Geometry check sheet. Reference: the model listing, model coordinates, mm. A direction names the side the tool comes from. Give positions to 0.01 mm unless a question says otherwise; leave off trailing zeros. Write each loop counter-clockwise with the first axis right and the second up, starting at its lowest first coordinate (ties: lowest second). Pieces come first, ordered by that corner, then holes.
(1) Cross-section at C-C (x = 43). Record the boundary of the cut face in (y, z), and give its area (3 significant figures).
(2) Depth check by flat-ended pin: P1, Ø2, axis at y = 2, z = -41, coming from the -X side; P2, Ø5, axis at x = 64.5, z = -31.5, coming from the -Y side; P3, Ø4, axis at x = 79, z = 45, coming from the -Y side; P4, Ø3.5, axis at x = -79, z = -45.5, coming from the +Y side. Enter the tip coordinate at first touch or a pass-through.
(3) Tool access check on faces 1 (the cylindrical face through (75, 1, 42)), 2 (the cylindrical face through (79.46, 2.92, -48.47)), 3 (the cylindrical face through (-77.3, 0.64, 45.07)). Record the directions out of +Z, -Z, +X, -X, +Y, -Y that give a thin tool (end or side, any length) a straight path to the whole face; none if there is none.
(4) Mould release check, pull along X, two halves, no side actions. Record for faces 4 (the flat face through (-77, 1.3, 46)), 5 (the flat face through (-84, 2, -34)), 6 (the flat face through (1, 2, -50)), 7 (the flat face through (84, 2, -34)): +X half, -X half, draft (parallel to the pull), parting line (faces both ways), or undercut.
(5) Cross-section at B-B (z = -6). Record the boundary of the cut face in (x, y), and give its area (3 significant figures).
(6) Thickness scan on line 1 along Z through (x, y) = (79, 2.6); line 2 along X through (y, z) = (2.9, -45); line 3 along Z through (x, y) = (9, 1.45). Record the ranges inside material, lowest first.
(7) Cross-section at A-A (y = 3.5). Record the boundary of the cut face in (x, z).
```python
from build123d import *

# Parameters (mm, degrees)
SKIZZE1_W                                            = 89
SKIZZE1_H                                            = 50
AUFSATZ_LINEAR_AUSTRAGEN1_DEPTH                      = 4.5
SKIZZE3_W                                            = 16
SKIZZE3_H                                            = 12
SCHNITT_LINEAR_AUSTRAGEN2_DEPTH                      = 5.5
VERRUNDUNG1_R                                        = 2
LINEARES_MUSTER1_COUNT                               = 3
LINEARES_MUSTER1_PITCH                               = 16
LINEARES_MUSTER1_COUNT_DIR2                          = 4
LINEARES_MUSTER1_PITCH_DIR2                          = 20
VERRUNDUNG1_OF_LINEARES_MUSTER1_R                    = 2
SKIZZE2_R                                            = 5
AUFSATZ_LINEAR_AUSTRAGEN2_DEPTH                      = 4.5
STIRNSENKUNG_F_R_M3_FLACHKOPFSCHRAUBE_MI_D           = 3.4
STIRNSENKUNG_F_R_M3_FLACHKOPFSCHRAUBE_MI_CBORE_D     = 7
STIRNSENKUNG_F_R_M3_FLACHKOPFSCHRAUBE_MI_CBORE_DEPTH = 3.2
VERRUNDUNG3_R                                        = 3
SCHNITT_LINEAR_AUSTRAGEN3_DEPTH                      = 1.5
AUFSATZ_LINEAR_AUSTRAGEN3_DEPTH                      = 3
SKIZZE8_W                                            = 10
SKIZZE8_H                                            = 35
SCHNITT_LINEAR_AUSTRAGEN4_DEPTH                      = 5.5
VERRUNDUNG4_R                                        = 2


with BuildPart() as part:
    # Skizze1 → Aufsatz-Linear austragen1 (new body)
    with BuildSketch(Plane(origin=(0, 0, 0), x_dir=(1, 0, 0), z_dir=(0, 1, 0))):
        with Locations((-44.5, 25)):
            Rectangle(SKIZZE1_W, SKIZZE1_H)
    extrude(amount=AUFSATZ_LINEAR_AUSTRAGEN1_DEPTH)

    # Skizze3 → Schnitt-Linear austragen2 (cut, through all)
    with BuildSketch(Plane(origin=(0, 4.5, 0), x_dir=(1, 0, 0), z_dir=(0, 1, 0))):
        with Locations((-11, 9)):
            Rectangle(SKIZZE3_W, SKIZZE3_H)
    schnitt_linear_austragen2 = extrude(amount=-SCHNITT_LINEAR_AUSTRAGEN2_DEPTH, mode=Mode.SUBTRACT)

    # Verrundung1
    verrundung1_edges = [part.edges().sort_by_distance(p)[0] for p in [
        (-3, 2.25, -15),
        (-3, 2.25, -3),
        (-19, 2.25, -3),
        (-19, 2.25, -15),
    ]]
    fillet(verrundung1_edges, radius=VERRUNDUNG1_R)

    # Lineares Muster1: Schnitt-Linear austragen2 3 × 4
    with Locations(*[(-j * LINEARES_MUSTER1_PITCH_DIR2, 0, -i * LINEARES_MUSTER1_PITCH) for i in range(LINEARES_MUSTER1_COUNT) for j in range(LINEARES_MUSTER1_COUNT_DIR2) if (i, j) != (0, 0)]):
        add(schnitt_linear_austragen2, mode=Mode.SUBTRACT)

    # Verrundung1 of Lineares Muster1
    verrundung1_of_lineares_muster1_edges = [part.edges().sort_by_distance(p)[0] for p in [
        (-23, 2.25, -15),
        (-23, 2.25, -3),
        (-39, 2.25, -3),
        (-39, 2.25, -15),
        (-43, 2.25, -15),
        (-43, 2.25, -3),
        (-59, 2.25, -3),
        (-59, 2.25, -15),
        (-63, 2.25, -15),
        (-63, 2.25, -3),
        (-79, 2.25, -3),
        (-79, 2.25, -15),
        (-3, 2.25, -31),
        (-3, 2.25, -19),
        (-19, 2.25, -19),
        (-19, 2.25, -31),
        (-23, 2.25, -31),
        (-23, 2.25, -19),
        (-39, 2.25, -19),
        (-39, 2.25, -31),
        (-43, 2.25, -31),
        (-43, 2.25, -19),
        (-59, 2.25, -19),
        (-59, 2.25, -31),
        (-63, 2.25, -31),
        (-63, 2.25, -19),
        (-79, 2.25, -19),
        (-79, 2.25, -31),
        (-3, 2.25, -47),
        (-3, 2.25, -35),
        (-19, 2.25, -35),
        (-19, 2.25, -47),
        (-23, 2.25, -47),
        (-23, 2.25, -35),
        (-39, 2.25, -35),
        (-39, 2.25, -47),
        (-43, 2.25, -47),
        (-43, 2.25, -35),
        (-59, 2.25, -35),
        (-59, 2.25, -47),
        (-63, 2.25, -47),
        (-63, 2.25, -35),
        (-79, 2.25, -35),
        (-79, 2.25, -47),
    ]]
    fillet(verrundung1_of_lineares_muster1_edges, radius=VERRUNDUNG1_OF_LINEARES_MUSTER1_R)

    # Skizze2 → Aufsatz-Linear austragen2 (add)
    with BuildSketch(Plane(origin=(0, 4.5, 0), x_dir=(1, 0, 0), z_dir=(0, 1, 0))):
        with Locations((-79, 45)):
            Circle(SKIZZE2_R)
    extrude(amount=-AUFSATZ_LINEAR_AUSTRAGEN2_DEPTH)

    # Stirnsenkung für M3 Flachkopfschraube mit Schlitz1 (through all)
    with Locations(Plane(origin=(0, 4.5, 0), x_dir=(1, 0, 0), z_dir=(0, 1, 0))):
        with Locations((-79, 45)):
            CounterBoreHole(STIRNSENKUNG_F_R_M3_FLACHKOPFSCHRAUBE_MI_D / 2, STIRNSENKUNG_F_R_M3_FLACHKOPFSCHRAUBE_MI_CBORE_D / 2, STIRNSENKUNG_F_R_M3_FLACHKOPFSCHRAUBE_MI_CBORE_DEPTH)

    # Verrundung3
    verrundung3_edges = [part.edges().sort_by_distance(p)[0] for p in [
        (-74.417424305, 2.25, -47),
        (-79, 2.25, -40),
    ]]
    fillet(verrundung3_edges, radius=VERRUNDUNG3_R)

    # Skizze6 → Schnitt-Linear austragen3 (cut)
    with BuildSketch(Plane.XZ):
        Polygon((0, 0), (-79, 0), (-79, -37), (-71.062746067, -37), (-71.062746067, -47), (0, -47), align=None)
    extrude(amount=-SCHNITT_LINEAR_AUSTRAGEN3_DEPTH, mode=Mode.SUBTRACT)

    # Skizze7 → Aufsatz-Linear austragen3 (add)
    with BuildSketch(Plane.XZ.offset(-1.5)):
        with BuildLine():
            Line((-79, 0), (0, 0))
            Line((0, 0), (0, -47))
            Line((0, -47), (-71.062746067, -47))
            ThreePointArc((-71.062746067, -47), (-73.04705955, -46.25), (-74.039216292, -44.375))
            ThreePointArc((-74.039216292, -44.375), (-75.037392467, -41.950780175), (-77.125, -40.364875946))
            ThreePointArc((-77.125, -40.364875946), (-78.487468593, -39.260852496), (-79, -37.583801513))
            Line((-79, -37.583801513), (-79, 0))
        make_face()
    extrude(amount=-AUFSATZ_LINEAR_AUSTRAGEN3_DEPTH)

    # Spiegeln1: part across plane


with BuildPart() as part_1:
    add(part.part)
    add(part.part.mirror(Plane(origin=(0, 4.5, 0), x_dir=(1, 0, 0), z_dir=(0, 0, -1))))

    # Skizze8 → Schnitt-Linear austragen4 (cut, through all)
    with BuildSketch(Plane.XZ):
        with Locations((-89, -32.5)):
            Rectangle(SKIZZE8_W, SKIZZE8_H)
    extrude(amount=-SCHNITT_LINEAR_AUSTRAGEN4_DEPTH, mode=Mode.SUBTRACT)

    # Verrundung4
    verrundung4_edges = [part_1.edges().sort_by_distance(p)[0] for p in [
        (-84, 2.25, -15),
    ]]
    fillet(verrundung4_edges, radius=VERRUNDUNG4_R)

    # Spiegeln2: part across plane


with BuildPart() as part_2:
    add(part_1.part)
    add(part_1.part.mirror(Plane(origin=(0, 4.5, 0), x_dir=(0, 0, 1), z_dir=(-1, 0, 0))))


solid = part_2.part
```
Reply:
1. outline: (0, -50) - (4.5, -50) - (4.5, 50) - (0, 50) - (0, 47) - (1.5, 47) - (1.5, -47) - (0, -47) - close
1. area: 309 mm2
2. P1: stops at x = -84
2. P2: stops at y = 1.5
2. P3: stops at y = 0
2. P4: stops at y = 1.3
3. face 1: -Y
3. face 2: +Y
3. face 3: +Y, -Y
4. face 4: undercut
4. face 5: -X half
4. face 6: draft
4. face 7: +X half
5. outline: (-89, 0) - (-79, 0) - (-79, 1.5) - (79, 1.5) - (79, 0) - (89, 0) - (89, 4.5) - (-89, 4.5) - close
5. area: 564 mm2
6. line 1: z = -50 to -48.5, -41.5 to 41.5, 48.5 to 50
6. line 2: x = -84 to -82.5, -75.5 to 75.5, 82.5 to 84
6. line 3: z = -50 to -47, 47 to 50
7. outline: (-89, -15) - (-86, -15) arc R2 cw to (-84, -17) - (-84, -50) - (84, -50) - (84, -17) arc R2 cw to (86, -15) - (89, -15) - (89, 50) - (-89, 50) - close; hole circle Ø7 at (-79, -45); hole circle Ø7 at (-79, 45); hole circle Ø7 at (79, -45); hole circle Ø7 at (79, 45)
